```python
from build123d import *

# Parameters (mm, degrees)
BOSS_EXTRUDE1_DEPTH             = 12.5
BOSS_EXTRUDE1_DEPTH_BACK        = 12.5
SKETCH3_R                       = 6.6
CUT_EXTRUDE1_DEPTH              = 42.688007868
TAP_DRILL_FOR_M3X0_5_TAP3_D     = 2.5
TAP_DRILL_FOR_M3X0_5_TAP3_DEPTH = 7
TAP_DRILL_FOR_M3X0_5_TAP3_TIP   = 0.751075774
TAP_DRILL_FOR_M4X0_7_TAP1_D     = 3.3
TAP_DRILL_FOR_M4X0_7_TAP1_DEPTH = 8
TAP_DRILL_FOR_M4X0_7_TAP1_TIP   = 0.991420021
TAP_DRILL_FOR_M3X0_5_TAP4_D     = 2.5
TAP_DRILL_FOR_M3X0_5_TAP4_DEPTH = 6.35
TAP_DRILL_FOR_M3X0_5_TAP5_D     = 2.5


with BuildPart() as part:
    # Sketch1 → Boss-Extrude1 (new, two sides: drawn at the far end of the back side and taken through both)
    with BuildSketch(Plane.XY.offset(-BOSS_EXTRUDE1_DEPTH_BACK)):
        Polygon((-14.6, 12.5), (-14.6, -27), (14.6, -27), (14.6, 12.5), (8.25, 12.5), (8.25, -19), (-8.25, -19), (-8.25, 12.5), align=None)
    extrude(amount=BOSS_EXTRUDE1_DEPTH + BOSS_EXTRUDE1_DEPTH_BACK)

    # Sketch3 → Cut-Extrude1 (cut, through all)
    with BuildSketch(Plane.ZY.offset(14.6)):
        with Locations(Location((0, 0, 0), (0, 0, 270))):
            Circle(SKETCH3_R)
    extrude(amount=-CUT_EXTRUDE1_DEPTH, mode=Mode.SUBTRACT)

    # Tap Drill for M3x0.5 Tap3
    with Locations(Plane(origin=(0, 12.5, 0), x_dir=(1, 0, 0), z_dir=(0, 1, 0))):
        with Locations((-11.425, 0), (11.425, 0)):
            Hole(TAP_DRILL_FOR_M3X0_5_TAP3_D / 2, depth=TAP_DRILL_FOR_M3X0_5_TAP3_DEPTH)
            with Locations((0, 0, -(TAP_DRILL_FOR_M3X0_5_TAP3_DEPTH + TAP_DRILL_FOR_M3X0_5_TAP3_TIP / 2))):  # 118° drill point
                Cone(0, TAP_DRILL_FOR_M3X0_5_TAP3_D / 2, TAP_DRILL_FOR_M3X0_5_TAP3_TIP, mode=Mode.SUBTRACT)

    # Tap Drill for M4x0.7 Tap1
    with Locations(Plane(origin=(0, -27, 0), x_dir=(-1, 0, 0), z_dir=(0, -1, 0))):
        with Locations((-10.1, 0), (10.1, 0)):
            Hole(TAP_DRILL_FOR_M4X0_7_TAP1_D / 2, depth=TAP_DRILL_FOR_M4X0_7_TAP1_DEPTH)
            with Locations((0, 0, -(TAP_DRILL_FOR_M4X0_7_TAP1_DEPTH + TAP_DRILL_FOR_M4X0_7_TAP1_TIP / 2))):  # 118° drill point
                Cone(0, TAP_DRILL_FOR_M4X0_7_TAP1_D / 2, TAP_DRILL_FOR_M4X0_7_TAP1_TIP, mode=Mode.SUBTRACT)

    # Tap Drill for M3x0.5 Tap4
    with Locations(Plane.ZY.offset(14.6)):
        with Locations((-9.53, 0), (9.53, 0)):
            Hole(TAP_DRILL_FOR_M3X0_5_TAP4_D / 2, depth=TAP_DRILL_FOR_M3X0_5_TAP4_DEPTH)

    # Tap Drill for M3x0.5 Tap5 (through all)
    with Locations(Plane(origin=(0, -27, 0), x_dir=(-1, 0, 0), z_dir=(0, -1, 0))):
        with Locations((0, -9.5), (0, 9.5)):
            Hole(TAP_DRILL_FOR_M3X0_5_TAP5_D / 2)


solid = part.part
```
Model file for the job. Use its own axes, mm. A direction names the side the tool comes from. Coordinates: 2 decimals unless noted, no trailing zeros. Order: outer loops, then holes, each group sorted by start corner. A loop starts at its lowest first (then second) coordinate and runs counter-clockwise, first axis right, second up. Notation, with made-up numbers: M -24.5,-4.5 L 26.5,-4.5 A15 ccw 26.5,9.5 Z; hole C 75.5,74 d3. An arc over 180 degrees is marked long. Answer as CSV lines item,"result".
(1) Flat gauge pins, fed straight in: pin 1 (12 mm diameter, centred on y = 0, z = 0, fed in from -X); pin 2 (3 mm diameter, centred on x = 0, z = 9.5, fed in from +Y); pin 3 (2 mm diameter, centred on y = 0, z = 9.53, fed in from -X); pin 4 (3 mm diameter, centred on x = 10.1, z = 0, fed in from -Y). Where does each tip first touch, or does it go through?
Geometry says:
pin 1,"passes through"
pin 2,"stops at y = -19"
pin 3,"stops at x = 8.25"
pin 4,"stops at y = -18.91"
(2) Band-saw the part on A-A, the plane x = 0. List the corners of the cut face in (y, z), then the cut area to 3 significant figures.
Geometry says:
outline,"M -27,-12.5 L -19,-12.5 L -19,-10.75 L -27,-10.75 Z; M -27,-8.25 L -19,-8.25 L -19,8.25 L -27,8.25 Z; M -27,10.75 L -19,10.75 L -19,12.5 L -27,12.5 Z"
area,"160 mm2"
(3) Band-saw the part on B-B, the plane y = -20. List the corners of the cut face in (x, z), then the cut area to 3 significant figures.
Geometry says:
outline,"M -14.6,-12.5 L 14.6,-12.5 L 14.6,12.5 L -14.6,12.5 Z; hole C -10.1,0 d3.3; hole C 0,-9.5 d2.5; hole C 0,9.5 d2.5; hole C 10.1,0 d3.3"
area,"703 mm2"
(4) 3-axis set-ups, long thin cutter, end or side, ignore diameter. For faces 4 (the cylindrical face through (-10.176, 9.448, -0.055)), 5 (the cylindrical face through (8.45, -22.94, -0.07)), 6 (the cylindrical face through (-11.381, 0.845, -8.609)), 7 (the cylindrical face through (-11.469, -6.097, -2.528)), 8 (the flat face through (-8.25, -7, 0)): which of +Z, -Z, +X, -X, +Y, -Y reach the whole face in a straight line?
Geometry says:
face 4,"+Y"
face 5,"-Y"
face 6,"-X"
face 7,"+X, -X"
face 8,"+Z, -Z, +Y"
(5) Band-saw the part on D-D, the plane x = 3. List the corners of the cut face in (y, z), then the cut area to 3 significant figures.
Geometry says:
outline,"M -27,-12.5 L -19,-12.5 L -19,12.5 L -27,12.5 Z"
area,"200 mm2"
(6) Pull direction Y, two halves, no side cores. Call faces 1 (the flat face through (0, -27, 0)), 2 (the cylindrical face through (10.27, 9.45, 0.48)), 3 (the cylindrical face through (11.381, -6.097, -2.528)): +Y half, -Y half, draft (parallel to the pull), parting line (faces both ways), or undercut.
Geometry says:
face 1,"-Y half"
face 2,"draft"
face 3,"undercut"
(7) Wall check: line 1 along X through (y, z) = (-2, 9.75); line 2 along Y through (x, z) = (-9.5, -9.53). Give the ranges that are in metal, low to high.
Geometry says:
line 1,"x = -14.6 to -8.25, 8.25 to 14.6"
line 2,"y = -27 to -1.25, 1.25 to 12.5"
(8) Band-saw the part on C-C, the plane z = 9. List the corners of the cut face in (x, y), then the cut area to 3 significant figures.
Geometry says:
outline,"M -14.6,-27 L -1.15,-27 L -1.15,-19 L -8.25,-19 L -8.25,-1.13 L -14.6,-1.13 Z; M -14.6,1.13 L -8.25,1.13 L -8.25,12.5 L -14.6,12.5 Z; M 1.15,-27 L 14.6,-27 L 14.6,12.5 L 8.25,12.5 L 8.25,-19 L 1.15,-19 Z"
area,"601 mm2"
